Input: part model. Units: mm. Frame: model coordinates. Round coordinates to 2 decimals unless told otherwise and drop trailing zeros. Order: outer loops, then holes, each group sorted by start corner. A loop starts at its lowest first (then second) coordinate and runs counter-clockwise, first axis right, second up.
Item 1: Cut plane A-A on z = 0. Output: boundary loops of the cut face in (x, y), then the cut area to 3 significant figures.
Item 2: Line query: L1, parallel to X at y = -1.25, z = 0; L2, parallel to Z at x = 69.85, y = 4.5; L3, parallel to X at y = 5.5, z = -1.25. Output: solid intervals per line, ascending.
Item 3: Cut plane B-B on x = 69.85. Output: boundary loops of the cut face in (y, z).
Item 4: Cut plane C-C on y = 8.75. Give the number of separate pieces and of enclosed holes in the cut face, then the cut area to 3 significant figures.
Item 5: First-contact query: pin 1 (3 mm diameter, centred on y = -6, z = -9, fed in from -X); pin 2 (1.5 mm diameter, centred on x = 13.5, y = 4.5, fed in from -Z); pin 3 (1 mm diameter, centred on x = 56.5, y = 8.5, fed in from -Z); pin 4 (1.5 mm diameter, centred on x = 22, y = 9.5, fed in from -Z). Flat tips, straight axial feed; report the tip coordinate or a pass-through.
Item 6: Cut plane D-D on x = 58.5. Output: boundary loops of the cut face in (y, z), then the cut area to 3 significant figures.
```python
from build123d import *
from OCP.BRepFilletAPI import BRepFilletAPI_MakeChamfer

# Parameters (mm, degrees)
SKETCH2_R               = 12.7
BOSS_EXTRUDE1_DEPTH     = 76.2
CHAMFER1_SIZE           = 2.54
CHAMFER1_SIZE2          = 1.466469684
CUT_EXTRUDE1_DEPTH      = 79.288057838
CUT_EXTRUDE1_DEPTH_BACK = 79.288057838
SKETCH6_R               = 1.5875


with BuildPart() as part:
    # Sketch2 → Boss-Extrude1 (new body)
    with BuildSketch(Plane(origin=(0, 0, 0), x_dir=(0, 0, -1), z_dir=(1, 0, 0))):
        with Locations(Location((0, 0, 0), (0, 0, 180))):
            Circle(SKETCH2_R)
    extrude(amount=BOSS_EXTRUDE1_DEPTH)

    # Chamfer1: one chamfer whose edges measure the first distance from different faces: ONE call of the kernel's chamfer builder (chamfer() names one face for all edges)
    chamfer1_edges_1 = [part.edges().sort_by_distance(p)[0] for p in [
        (0, 0, -12.7),
    ]]
    chamfer1_side_1 = [part.faces().sort_by_distance(p)[0] for p in [
        (0, 0, 0),
    ]]
    chamfer1_edges_2 = [part.edges().sort_by_distance(p)[0] for p in [
        (76.2, 0, -12.7),
    ]]
    chamfer1_side_2 = [part.faces().sort_by_distance(p)[0] for p in [
        (38.1, 0, -12.7),
    ]]
    chamfer1 = BRepFilletAPI_MakeChamfer(part.part.solid().wrapped)
    for e in chamfer1_edges_1:
        chamfer1.Add(CHAMFER1_SIZE, CHAMFER1_SIZE2, e.wrapped, chamfer1_side_1[0].wrapped)  # the first distance lies on this face
    for e in chamfer1_edges_2:
        chamfer1.Add(CHAMFER1_SIZE, CHAMFER1_SIZE2, e.wrapped, chamfer1_side_2[0].wrapped)  # the first distance lies on this face
    add(Compound.cast(chamfer1.Shape()), mode=Mode.REPLACE)

    # Sketch6 → Cut-Extrude1 (cut, two sides: drawn at the far end of the back side and taken through both)
    with BuildSketch(Plane(origin=(0, 0, 0), x_dir=(1, 0, 0), z_dir=(0, 1, 0)).offset(-CUT_EXTRUDE1_DEPTH_BACK)):
        with Locations(Location((6.35, 0, 0), (0, 0, 270))):
            Circle(SKETCH6_R)
        with Locations(Location((69.85, 0, 0), (0, 0, 270))):
            Circle(SKETCH6_R)
    extrude(amount=CUT_EXTRUDE1_DEPTH + CUT_EXTRUDE1_DEPTH_BACK, mode=Mode.SUBTRACT)


solid = part.part
```
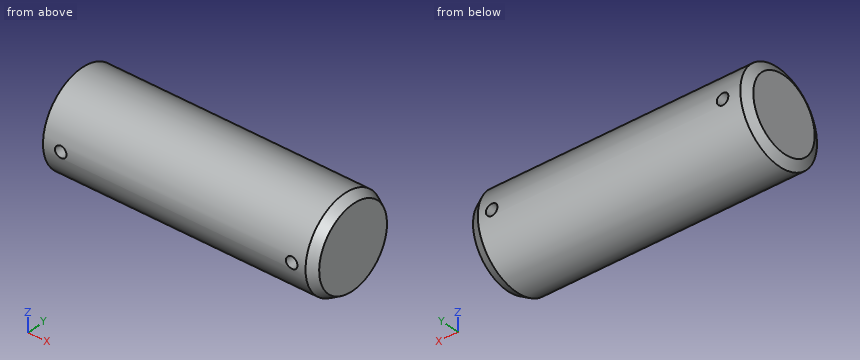
From the geometry:
1. outline: (0, -10.16) - (1.47, -12.7) - (4.76, -12.7) - (4.76, 12.7) - (1.47, 12.7) - (0, 10.16) - close; (7.94, -12.7) - (68.26, -12.7) - (68.26, 12.7) - (7.94, 12.7) - close; (71.44, -12.7) - (73.66, -12.7) - (76.2, -11.23) - (76.2, 11.23) - (73.66, 12.7) - (71.44, 12.7) - close
1. area: 1,770 mm2
2. L1: x = 0 to 4.76, 7.94 to 68.26, 71.44 to 76.2
2. L2: z = -11.88 to -1.59, 1.59 to 11.88
2. L3: x = 0 to 5.37, 7.33 to 68.87, 70.83 to 76.2
3. outline: (-12.6, -1.59) arc R12.7 ccw to (12.6, -1.59) - close; (-12.6, 1.59) - (12.6, 1.59) arc R12.7 ccw to start
4. separate pieces: 1
4. enclosed holes: 2
4. area: 1,380 mm2
5. pin 1: stops at x = 0
5. pin 2: stops at z = -12.13
5. pin 3: stops at z = -9.86
5. pin 4: stops at z = -9.2
6. outline: circle Ø25.4 at (0, 0)
6. area: 507 mm2
